The model under review builds one solid part; all positions refer to its coordinate system, in mm. Face numbers are marked on the shaded views. Round coordinates to 2 decimals unless told otherwise and drop trailing zeros. Loops run counter-clockwise (first coordinate to the right, second up) from the corner with the lowest first, then second, coordinate; pieces in that order, holes last. Notation, with made-up numbers: M 64.5,7 L 114.5,7 A8 cw 114.5,22 Z; hole C -38.75,44 d2. An arc over 180 degrees is marked long. One line per question, with ' | ' between items.
from build123d import *

# Parameters (mm, degrees)
F1_DEPTH = 13
F2_R     = 5
F3_R     = 1
F4_W     = 7
F4_H     = 80.0645950389
F5_DEPTH = 10


with BuildPart() as f1:
    # F0 (on Right) → F1 (new body)
    with BuildSketch(Plane.YZ):
        Polygon((-56.8815148667, 19.1431619976), (-69.8815148667, 19.1431619976), (-69.8815148667, -60.8568380024), (-56.8815148667, -60.8568380024), (-56.8815148667, -47.8568380024), align=None)
    extrude(amount=F1_DEPTH)

    # F2
    f2_edges = [f1.edges().sort_by_distance(p)[0] for p in [
        (6.5, -56.881515, 19.143162),
    ]]
    fillet(f2_edges, radius=F2_R)

    # F3
    f3_edges = [f1.edges().sort_by_distance(p)[0] for p in [
        (0, -56.881515, -23.356838),
        (13, -56.881515, -23.356838),
        (0, -65.881515, 19.143162),
        (13, -65.881515, 19.143162),
        (0, -58.345981, 17.678696),
        (13, -58.345981, 17.678696),
    ]]
    fillet(f3_edges, radius=F3_R)

    # F4 (on face) → F5 (cut)
    with BuildSketch(Plane(origin=(0, -56.8815148667, 0), x_dir=(-1, 0, 0), z_dir=(0, 1, 0))):
        with Locations((-6.5, -20.824540483)):
            Rectangle(F4_W, F4_H)
    extrude(amount=-F5_DEPTH, mode=Mode.SUBTRACT)


solid = f1.part
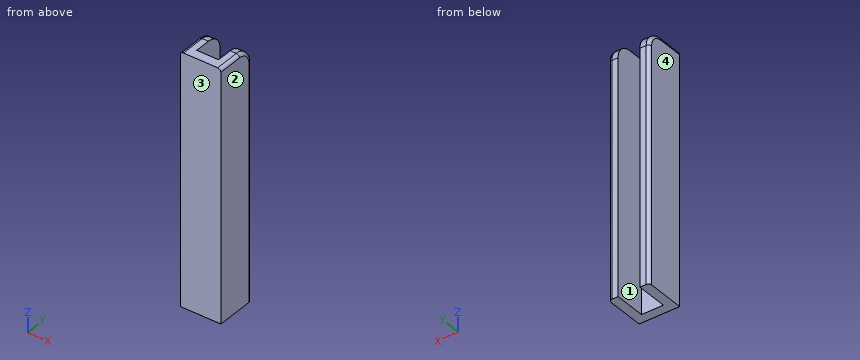
1) Add section A-A on y = -64.25. State the section outline as (x, z) points.
Output values:
outline: M 0,-60.86 L 3,-60.86 L 3,19.14 L 1,19.14 A1 ccw 0,18.14 Z; M 10,-60.86 L 13,-60.86 L 13,18.14 A1 ccw 12,19.14 L 10,19.14 Z
2) Insertion check: P1, Ø5.5, axis at x = 7, z = -37.5, coming from the +Y side. The pin has a flat end and moves straight along its axis. Give the tip position at first contact, or say it passes through.
Output values:
P1: stops at y = -66.88
3) Add section B-B on z = -5. State the section outline as (x, y) points, then the cut area to 3 significant figures.
Output values:
outline: M 0,-69.88 L 13,-69.88 L 13,-57.88 A1 ccw 12,-56.88 L 10,-56.88 L 10,-66.88 L 3,-66.88 L 3,-56.88 L 1,-56.88 A1 ccw 0,-57.88 Z | area: 98.6 mm²
4) Add section C-C on x = 8.5. State the section outline as (y, z) points.
Output values:
outline: M -69.88,-60.86 L -66.88,-60.86 L -66.88,19.14 L -69.88,19.14 Z
5) Mouldability with a two-part tool opening along X and no side actions: class the marked faces 1, 2, 3 and 4 as +X half, -X half, draft (parallel to the pull), parting line (faces both ways), or undercut.
Output values:
face 1: undercut | face 2: +X half | face 3: draft | face 4: -X half
6) For line 1 (X direction, y = -62.5, z = -34); line 2 (Y direction, x = 5, z = -26); line 3 (X direction, y = -57.5, z = -20), list the stretches that pass through material, from the lowest coordinate up.
Output values:
line 1: x = 0 to 3, 10 to 13 | line 2: y = -69.88 to -66.88 | line 3: x = 0.08 to 3, 10 to 12.92
